Part model, mm, in its own coordinate system. Give positions to 0.01 mm unless a question says otherwise; leave off trailing zeros. Write each loop counter-clockwise with the first axis right and the second up, starting at its lowest first coordinate (ties: lowest second). Pieces come first, ordered by that corner, then holes. Notation, with made-up numbers: M 61,0 L 112,0 A30 ccw 112,33 Z; hole C 32.5,47 d6. An arc over 180 degrees is marked long. Answer as CSV lines item,"result". Start each with the question number.
Item 1: Band-saw the part on B-B, the plane z = 119. List the corners of the cut face in (x, y).
Item 2: Pin check, flat tips, straight feed: pin 1 (0.9 mm diameter, centred on x = 1, y = 27.5, fed in from +Z); pin 2 (1.5 mm diameter, centred on x = 1.5, z = -3.5, fed in from +Y). Stop position of each tip, or through.
Item 3: Wall check: L1, parallel to Z at x = 1.5, y = 52. Give the ranges that are in metal, low to high. Write a range as from..to.
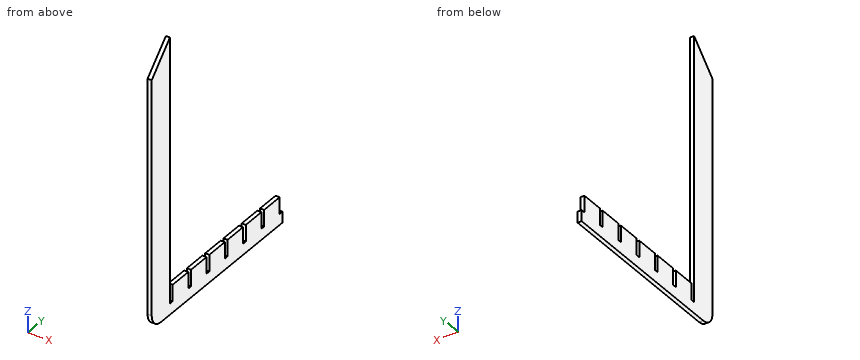
from build123d import *

# Parameters (mm, degrees)
SKETCH1_W           = 20
SKETCH1_H           = 123
BOSS_EXTRUDE1_DEPTH = 3
SKETCH2_W           = 12
SKETCH2_H           = 3
CUT_EXTRUDE1_DEPTH  = 125.651514231
LPATTERN1_COUNT     = 7
LPATTERN1_PITCH     = 20
BOSS_EXTRUDE2_DEPTH = 3
FILLET1_R           = 10


with BuildPart() as part:
    # Sketch1 → Boss-Extrude1 (new body)
    with BuildSketch(Plane(origin=(0, 0, 0), x_dir=(0, 0, -1), z_dir=(1, 0, 0))):
        with Locations((10, 61.5)):
            Rectangle(SKETCH1_W, SKETCH1_H)
    extrude(amount=BOSS_EXTRUDE1_DEPTH)

    # Sketch2 → Cut-Extrude1 (cut, through all)
    with BuildSketch(Plane(origin=(3, 0, 0), x_dir=(0, 0, -1), z_dir=(1, 0, 0))):
        with Locations((6, 1.5)):
            Rectangle(SKETCH2_W, SKETCH2_H)
    cut_extrude1 = extrude(amount=-CUT_EXTRUDE1_DEPTH, mode=Mode.SUBTRACT)

    # LPattern1: Cut-Extrude1 ×7
    with Locations(*[(0, i * LPATTERN1_PITCH, 0) for i in range(1, LPATTERN1_COUNT)]):
        add(cut_extrude1, mode=Mode.SUBTRACT)

    # Sketch3 → Boss-Extrude2 (add)
    with BuildSketch(Plane.ZY):
        Polygon((180, 0), (160, -20), (-20, -20), (-20, 0), align=None)
    extrude(amount=-BOSS_EXTRUDE2_DEPTH)

    # Fillet1
    fillet1_edges = [part.edges().sort_by_distance(p)[0] for p in [
        (1.5, -20, -20),
    ]]
    fillet(fillet1_edges, radius=FILLET1_R)


solid = part.part
Output:
1,outline,"M 0,-20 L 3,-20 L 3,0 L 0,0 Z"
2,pin 1,"z = 0"
2,pin 2,"y = 120"
3,L1,"-20..0"
